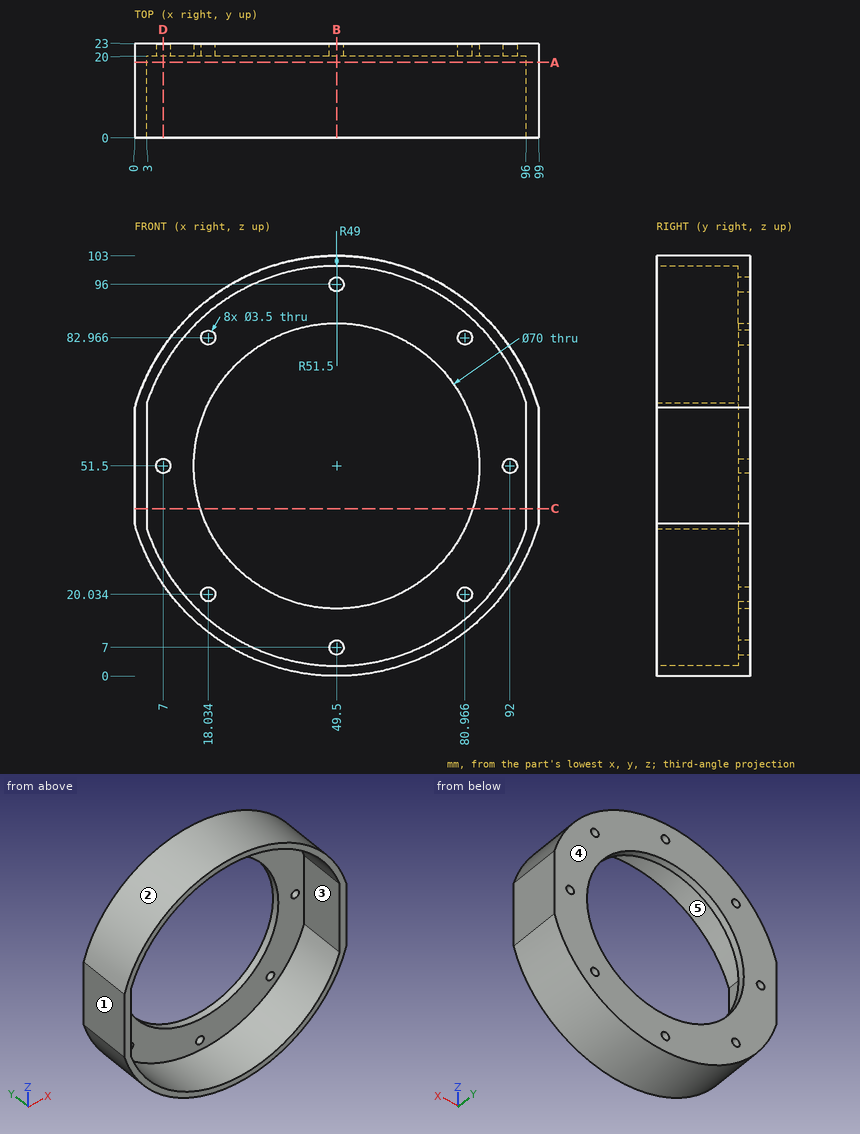
Answer from the drawing. Dimensions are ordinates in mm from the lowest x, y and z of the part. A direction names the side the tool comes from. Coordinates: 2 decimals unless noted, no trailing zeros. Write each loop counter-clockwise with the first axis right and the second up, starting at its lowest first coordinate (ties: lowest second). Pieces come first, ordered by that corner, then holes. Notation, with made-up numbers: M 49.5,-27.5 L 62.5,-27.5 A20 ccw 62.5,-9.5 Z; hole C 15.25,-8 d4. An arc over 180 degrees is marked long. Use one line per item in the form item = value. Start each with the question number.
1. A tool of negligible diameter and unlimited length cuts with its end or side. For the marked faces 4 and 5, from which of +Z, -Z, +X, -X, +Y, -Y can it reach the whole face along a straight path? Write none if from no direction.
2. Each of these flat-tipped pins is pushed along its axis until it touches: P1, Ø5, axis at x = 12.5, y = 20.5, coming from the -Z side; P2, Ø3, axis at x = 72.5, y = 5.5, coming from the +Z side; P3, Ø5.5, axis at x = 80.97, z = 82.97, coming from the -Y side; P4, Ø3, axis at x = 92, z = 51.5, coming from the -Y side. Where does it stop, or does it pass through?
3. The part is cut by section C-C (z = 41). Give the vertices of the cut face in (x, y), plus the area to 3 significant figures.
4. Straight lines are drawn through the part: probe 1 along X at (y, z) = (21.2, 51.5); probe 2 along X at (y, z) = (18, 54.5); probe 3 along X at (y, z) = (13, 91) (1 decimal). For each, find the intervals that lie inside material, in ascending order. Write a range as from..to.
5. The part is cut by section B-B (x = 49.5). Give the vertices of the cut face in (y, z).
6. The mould has two halves that part along Z. Classify the marked faces 1, 2 and 3: released by +Z, released by -Z, zero draft, split by the parting line, or undercut.
7. The part is cut by section A-A (y = 18.5). Give the vertices of the cut face in (x, z).
8. The part is cut by section D-D (x = 7). Give the vertices of the cut face in (y, z), plus the area to 3 significant figures.
Evaluation:
q1.face_4 = +Z, -Z, +X, -X, +Y
q1.face_5 = -Y
q2.P1 = 13.26
q2.P2 = 98.3
q2.P3 = 20
q2.P4 = through
q3.outline = M 0,0 L 3,0 L 3,20 L 16.11,20 L 16.11,23 L 0,23 Z; M 82.89,20 L 96,20 L 96,0 L 99,0 L 99,23 L 82.89,23 Z
q3.area = 217 mm^2
q4.probe_1 = 0..5.25, 8.75..14.5, 84.5..90.25, 93.75..99
q4.probe_2 = 0..3, 96..99
q4.probe_3 = 16.5..20.5, 78.5..82.5
q5.outline = M 0,0 L 23,0 L 23,5.25 L 20,5.25 L 20,2.5 L 0,2.5 Z; M 0,100.5 L 20,100.5 L 20,97.75 L 23,97.75 L 23,103 L 0,103 Z; M 20,8.75 L 23,8.75 L 23,16.5 L 20,16.5 Z; M 20,86.5 L 23,86.5 L 23,94.25 L 20,94.25 Z
q6.face_1 = zero draft
q6.face_2 = released by +Z
q6.face_3 = undercut
q7.outline = M 0,37.29 A51.5 ccw 99,37.29 L 99,65.71 A51.5 ccw 0,65.71 Z; hole M 3,36.05 A49 ccw 96,36.05 L 96,66.95 A49 ccw 3,66.95 Z
q8.outline = M 0,22.41 L 23,22.41 L 23,49.75 L 20,49.75 L 20,27.11 L 0,27.11 Z; M 0,75.89 L 20,75.89 L 20,53.25 L 23,53.25 L 23,80.59 L 0,80.59 Z
q8.area = 352 mm^2
